```python
from build123d import *

# Parameters (mm, degrees)
F0_W         = 6
F0_H         = 18
F1_DEPTH     = 8
F3_DEPTH     = 18
F4_DEPTH     = 6
F5_DEPTH     = 4.2
F10_DEPTH    = 6
F11_R        = 2.25
F13_DEPTH    = 25
F14_W        = 4
F14_H        = 4.5
F15_DEPTH    = 25
F16_W        = 2.5
F16_H        = 17.5837995484
F16_W_2      = 3.5
F17_DEPTH    = 18.001
F18_W        = 2
F18_H        = 6
F19_DEPTH    = 30
F21_DEPTH    = 6
F23_DEPTH    = 3.75
F24_R        = 3
F26_DEPTH    = 25
F27_DEPTH    = 2
F28_T1_DEPTH = 16.2867319519
F30_DEPTH    = 6
F31_T1_DEPTH = 9.0166310888
F33_DEPTH    = 6


# Not quite as in the source:
# - a fillet or chamfer that OpenCascade refuses, or shapes differently, is made with other operations: its cross-section is extruded or revolved along the edge and cut away or added


with BuildPart() as f1:
    # F0 (on Right) → F1 (new body)
    with BuildSketch(Plane.YZ):
        with Locations((-22.1395939865, -6.3859075308)):
            Rectangle(F0_W, F0_H)
    extrude(amount=F1_DEPTH)


with BuildPart() as f3:
    # F2 (on face) → F3 (new body)
    with BuildSketch(Plane.XZ.offset(25.1395939865)):
        with BuildLine():
            ThreePointArc((4, -15.3859075308), (1.0655068581, -22.4704006727), (8.15, -19.5359075308))
            ThreePointArc((8.15, -19.5359075308), (6.9344931419, -16.6014143889), (4, -15.3859075308))
        make_face()
    extrude(amount=F3_DEPTH)


with BuildPart() as f4:
    # F4 (new, through all): a face of the model
    f4_faces = [f3.part.faces().sort_by_distance(p)[0] for p in [
        (4, -25.1395939865, -19.5359075308),
    ]]
    extrude(f4_faces, amount=F4_DEPTH)


with BuildPart() as f5:
    # F5 (new): a face of the model
    f5_faces = [f1.part.faces().sort_by_distance(p)[0] for p in [
        (4, -22.1395939865, -15.3859075308),
    ]]
    extrude(f5_faces, amount=F5_DEPTH)


with BuildPart() as f3_1:
    add(f3.part)

    # F6: union F4, F5, F1
    add(f4.part)
    add(f5.part)
    add(f1.part)

    # F8 (on mid) → F9 (revolve)
    with BuildSketch(Plane.YZ.offset(4)):
        Polygon((-43.1395939865, -15.3859075308), (-39.6395939865, -15.3859075308), (-39.6395939865, -14.6359075308), (-40.6395939865, -14.6359075308), align=None)
    revolve(axis=Axis((4, -25.1395939865, -19.5359075308), (0, 1, 0)))


with BuildPart() as f10:
    # F10 (new): a face of the model
    f10_faces = [f3_1.part.faces().sort_by_distance(p)[0] for p in [
        (4, -22.1395939865, 2.6140924692),
    ]]
    extrude(f10_faces, amount=F10_DEPTH)

    # F12: union F3
    add(f3_1.part)

    # F11 (on face) → F13 (cut)
    with BuildSketch(Plane(origin=(0, -19.1395939865, 0), x_dir=(-1, 0, 0), z_dir=(0, 1, 0))):
        with Locations((-4, 5.1140924692)):
            Circle(F11_R)
    extrude(amount=-F13_DEPTH, mode=Mode.SUBTRACT)

    # F14 (on face) → F15 (cut)
    with BuildSketch(Plane(origin=(0, -19.1395939865, 0), x_dir=(-1, 0, 0), z_dir=(0, 1, 0))):
        with Locations((-4, 7.3640924692)):
            Rectangle(F14_W, F14_H)
    extrude(amount=-F15_DEPTH, mode=Mode.SUBTRACT)

    # F16 (on face) → F17 (cut, through all)
    with BuildSketch(Plane.XZ.offset(25.1395939865)):
        with Locations((-0.75, -18.0519367568)):
            Rectangle(F16_W, F16_H)
        with Locations((9.25, -18.0519367568)):
            Rectangle(F16_W_2, F16_H)
    extrude(amount=F17_DEPTH, mode=Mode.SUBTRACT)

    # F18 (on face) → F19 (join)
    with BuildSketch(Plane.XY.offset(8.6140924692)):
        with Locations((-1, -22.1395939865)):
            Rectangle(F18_W, F18_H)
        with Locations((9, -22.1395939865)):
            Rectangle(F18_W, F18_H)
    extrude(amount=-F19_DEPTH)

    # F20 (on face) → F21 (join, through all)
    with BuildSketch(Plane(origin=(0, -19.1395939865, 0), x_dir=(-1, 0, 0), z_dir=(0, 1, 0))):
        with BuildLine():
            Line((-8, -21.3859075308), (-10, -21.3859075308))
            Line((-10, -21.3859075308), (-10, -23.6859075308))
            Line((-10, -23.6859075308), (-4, -23.6859075308))
            ThreePointArc((-4, -23.6859075308), (-6.5133623932, -22.8382566159), (-8, -20.6415747502))
            Line((-8, -20.6415747502), (-8, -21.3859075308))
        make_face()
        with BuildLine():
            Line((2, -23.6859075308), (2, -21.3859075308))
            Line((2, -21.3859075308), (0, -21.3859075308))
            Line((0, -21.3859075308), (0, -20.6415747502))
            ThreePointArc((0, -20.6415747502), (-1.4866376068, -22.8382566159), (-4, -23.6859075308))
            Line((-4, -23.6859075308), (2, -23.6859075308))
        make_face()
        with BuildLine():
            Line((2, -13.6859075308), (-10, -13.6859075308))
            Line((-10, -13.6859075308), (-10, -21.3859075308))
            Line((-10, -21.3859075308), (-8, -21.3859075308))
            Line((-8, -21.3859075308), (-8, -20.6415747502))
            ThreePointArc((-8, -20.6415747502), (-6.5133623932, -22.8382566159), (-4, -23.6859075308))
            ThreePointArc((-4, -23.6859075308), (-1.4866376068, -22.8382566159), (0, -20.6415747502))
            Line((0, -20.6415747502), (0, -21.3859075308))
            Line((0, -21.3859075308), (2, -21.3859075308))
            Line((2, -21.3859075308), (2, -13.6859075308))
        make_face()
    extrude(amount=-F21_DEPTH)

    # F22 (on face) → F23 (join)
    with BuildSketch(Plane.XZ.offset(25.1395939865)):
        with BuildLine():
            Line((10, -23.6859075308), (10, -12.8277035983))
            ThreePointArc((10, -12.8277035983), (4, -10.5359075308), (-2, -12.8277035983))
            Line((-2, -12.8277035983), (-2, -23.6859075308))
            Line((-2, -23.6859075308), (10, -23.6859075308))
        make_face()
    extrude(amount=F23_DEPTH)

    # F24
    f24_edges = [f10.edges().sort_by_distance(p)[0] for p in [
        (-2, -24.014594, -23.685908),
        (10, -24.014594, -23.685908),
    ]]
    fillet(f24_edges, radius=F24_R)

    # F25 (on face) → F26 (cut)
    with BuildSketch(Plane.XZ.offset(28.8895939865)):
        with BuildLine():
            ThreePointArc((-0.15, -19.5359075308), (4, -15.3859075308), (8.15, -19.5359075308))
            Line((8.15, -19.5359075308), (10, -19.5359075308))
            Line((10, -19.5359075308), (10, -10.5359075308))
            Line((10, -10.5359075308), (-2, -10.5359075308))
            Line((-2, -10.5359075308), (-2, -19.5359075308))
            Line((-2, -19.5359075308), (-0.15, -19.5359075308))
        make_face()
    extrude(amount=F26_DEPTH, mode=Mode.SUBTRACT)

    # F27 (add): faces of the model
    f27_faces = [f10.faces().sort_by_distance(p)[0] for p in [
        (0, -22.1395939865, 8.6140924692),
        (8, -22.1395939865, 8.6140924692),
    ]]
    extrude(f27_faces, amount=F27_DEPTH)

    # F28: chamfer of 2 on 4 edges, made by hand

    # F28_s2 → F28_t1 (cut)
    with BuildSketch(Plane.XZ.offset(13.9962280105)):
        Polygon((8, 10.6140924692), (6, 8.6140924692), (6, 10.6140924692), align=None)
        Polygon((2, 8.6140924692), (0, 10.6140924692), (2, 10.6140924692), align=None)
    extrude(amount=F28_T1_DEPTH, mode=Mode.SUBTRACT)

    # F29 (on face) → F30 (join)
    with BuildSketch(Plane(origin=(0, -19.1395939865, 0), x_dir=(-1, 0, 0), z_dir=(0, 1, 0))):
        with BuildLine():
            Line((-6.0155644371, 6.1140924692), (-10, 6.1140924692))
            Line((-10, 6.1140924692), (-10, -20.6859075308))
            ThreePointArc((-10, -20.6859075308), (-9.1213203436, -22.8072278743), (-7, -23.6859075308))
            Line((-7, -23.6859075308), (-1, -23.6859075308))
            ThreePointArc((-1, -23.6859075308), (1.1213203436, -22.8072278743), (2, -20.6859075308))
            Line((2, -20.6859075308), (2, 6.1140924692))
            Line((2, 6.1140924692), (-1.9844355629, 6.1140924692))
            ThreePointArc((-1.9844355629, 6.1140924692), (-4, 2.8640924692), (-6.0155644371, 6.1140924692))
        make_face()
    extrude(amount=F30_DEPTH)

    # F31: chamfer of 1.5 on 2 edges, made by hand

    # F31_s2 → F31_t1 (cut)
    with BuildSketch(Plane.XZ.offset(10.1229628977)):
        with BuildLine():
            Line((7.2214544106, 6.1569815348), (6.2075003037, 5.1205433408))
            Line((6.2075003037, 5.1205433408), (6.1775075177, 5.119885475))
            ThreePointArc((6.1775075177, 5.119885475), (6.1595192188, 5.6287542453), (5.9886902446, 6.1007591359))
            Line((5.9886902446, 6.1007591359), (6.0155644371, 6.1440924692))
            ThreePointArc((6.0155644371, 6.1440924692), (6.6185094238, 6.1440924692), (7.2214544106, 6.1869815348))
            Line((7.2214544106, 6.1869815348), (7.2214544106, 6.1569815348))
        make_face()
        with BuildLine():
            Line((0.7785455894, 6.1569815348), (1.7924996963, 5.1205433408))
            Line((1.7924996963, 5.1205433408), (1.8224924823, 5.119885475))
            ThreePointArc((1.8224924823, 5.119885475), (1.8404807812, 5.6287542453), (2.0113097554, 6.1007591359))
            Line((2.0113097554, 6.1007591359), (1.9844355629, 6.1440924692))
            ThreePointArc((1.9844355629, 6.1440924692), (1.3814905762, 6.1440924692), (0.7785455894, 6.1869815348))
            Line((0.7785455894, 6.1869815348), (0.7785455894, 6.1569815348))
        make_face()
    extrude(amount=F31_T1_DEPTH, mode=Mode.SUBTRACT)

    # F32 (on face) → F33 (join)
    with BuildSketch(Plane(origin=(0, -13.1395939865, 0), x_dir=(-1, 0, 0), z_dir=(0, 1, 0))):
        with BuildLine():
            ThreePointArc((-2, 6.1448688756), (-1.8193396117, 5.668367014), (-1.7505410494, 5.1634324064))
            Line((-1.7505410494, 5.1634324064), (-0.8205042363, 6.1140924692))
            Line((-0.8205042363, 6.1140924692), (2, 6.1140924692))
            Line((2, 6.1140924692), (2, 10.6140924692))
            Line((2, 10.6140924692), (0, 10.6140924692))
            Line((0, 10.6140924692), (-2, 8.6140924692))
            Line((-2, 8.6140924692), (-2, 6.1448688756))
        make_face()
        with BuildLine():
            Line((-8, 10.6140924692), (-10, 10.6140924692))
            Line((-10, 10.6140924692), (-10, 6.1140924692))
            Line((-10, 6.1140924692), (-7.1794957637, 6.1140924692))
            Line((-7.1794957637, 6.1140924692), (-6.2494589506, 5.1634324064))
            ThreePointArc((-6.2494589506, 5.1634324064), (-6.1806603883, 5.668367014), (-6, 6.1448688756))
            Line((-6, 6.1448688756), (-6, 8.6140924692))
            Line((-6, 8.6140924692), (-8, 10.6140924692))
        make_face()
        with BuildLine():
            Line((-7.1794957637, 6.1140924692), (-10, 6.1140924692))
            Line((-10, 6.1140924692), (-10, -12.8277035983))
            Line((-10, -12.8277035983), (-10, -20.6859075308))
            ThreePointArc((-10, -20.6859075308), (-9.1213203436, -22.8072278743), (-7, -23.6859075308))
            Line((-7, -23.6859075308), (-1, -23.6859075308))
            ThreePointArc((-1, -23.6859075308), (1.1213203436, -22.8072278743), (2, -20.6859075308))
            Line((2, -20.6859075308), (2, -12.8277035983))
            Line((2, -12.8277035983), (2, 6.1140924692))
            Line((2, 6.1140924692), (-0.8205042363, 6.1140924692))
            Line((-0.8205042363, 6.1140924692), (-1.7505410494, 5.1634324064))
            ThreePointArc((-1.7505410494, 5.1634324064), (-4, 2.8640924692), (-6.2494589506, 5.1634324064))
            Line((-6.2494589506, 5.1634324064), (-7.1794957637, 6.1140924692))
        make_face()
    extrude(amount=F33_DEPTH)


solid = f10.part
```
Work out the finished part from the listing and answer in its coordinate system (mm). A direction names the side the tool comes from. Round coordinates to 2 decimals unless told otherwise and drop trailing zeros. Loops run counter-clockwise (first coordinate to the right, second up) from the corner with the lowest first, then second, coordinate; pieces in that order, holes last. Notation, with made-up numbers: M 40,-16.5 L 85,-16.5 A21 cw 85,2.5 Z; hole C -16,-39 d11. An arc over 180 degrees is marked long. Use CSV: the item, a comma, the result in double quotes.
Q1. Section A-A, the plane y = -11.5 is taken. Determine the outline of the cut face in (x, z).
Determined:
outline,"M -2,-20.69 A3 ccw 1,-23.69 L 7,-23.69 A3 ccw 10,-20.69 L 10,10.61 L 8,10.61 L 6,8.61 L 6,6.14 A2.25 cw long 2,6.14 L 2,8.61 L 0,10.61 L -2,10.61 Z"
Q2. Section B-B, the plane z = -3 is taken. Determine the outline of the cut face in (x, y), then the cut area to 3 significant figures.
Determined:
outline,"M -2,-25.14 L 10,-25.14 L 10,-7.14 L -2,-7.14 Z"
area,"216 mm2"
Q3. Section C-C, the plane y = -29.5 is taken. Determine the outline of the cut face in (x, z).
Determined:
outline,"M 0.5,-21.77 A4.15 ccw 7.5,-21.77 L 7.5,-17.31 A4.15 ccw 0.5,-17.31 Z"
Q4. Each of these flat-tipped pins is pushed along its axis until it touches: pin 1 (6 mm diameter, centred on x = 8.5, y = -14, fed in from -Z); pin 2 (1.5 mm diameter, centred on x = 2.5, z = 0.5, fed in from -Y); pin 3 (3 mm diameter, centred on x = -1, y = -16, fed in from +Z). Where does it stop, or does it pass through?
Determined:
pin 1,"z = -23.69"
pin 2,"y = -25.14"
pin 3,"z = 6.11"
Q5. The mould has two halves that part along Y. Classify faces 4 (the flat face through (4, -7.14, -6)), 5 (the flat face through (-1, -16, 6.114)), 6 (the flat face through (10, -16, -5)): pulls with the +Y half, pulls with the -Y half, needs draft (parallel to the pull), parting line crosses it, or undercut.
Determined:
face 4,"pulls with the +Y half"
face 5,"undercut"
face 6,"needs draft"
Q6. A tool of negligible diameter and unlimited length cuts with its end or side. For faces 1 (the cylindrical face through (4.055, -40.147, -24.436)), 2 (the flat face through (9, -16, 6.114)), 3 (the flat face through (1.014, -22.098, 9.6)), from which of +Z, -Z, +X, -X, +Y, -Y can it reach the whole face along a straight path? Write none if from no direction.
Determined:
face 1,"-Z, -Y"
face 2,"+Z, +X, -X"
face 3,"+Z, +Y, -Y"
Q7. Consider L1, parallel to X at y = -14, z = 5; L2, parallel to X at y = -13, z = 7; L3, parallel to Y at x = 0.75, z = -15. Determine where each line is inside the solid, lowest interval first.
Determined:
L1,"-2 to 1.75, 6.25 to 10"
L2,"-2 to 2, 6 to 10"
L3,"-28.89 to -7.14"
